```python
from build123d import *

# Parameters (mm, degrees)
SKETCH_1_R      = 2.5
EXTRUDE_1_DEPTH = 90


with BuildPart() as part:
    # 草图1 → 凸台-拉伸1 (new body)
    with BuildSketch(Plane(origin=(0, 0, 0), x_dir=(0, 0, -1), z_dir=(1, 0, 0))):
        with BuildLine():
            Line((10, 8.5), (10, 4))
            ThreePointArc((10, 4), (9.912132034, 3.787867966), (9.7, 3.7))
            ThreePointArc((9.7, 3.7), (9.487867966, 3.612132034), (9.4, 3.4))
            ThreePointArc((9.4, 3.4), (9.312132034, 3.187867966), (9.1, 3.1))
            Line((9.1, 3.1), (8.5, 3.1))
            ThreePointArc((8.5, 3.1), (8.287867966, 3.187867966), (8.2, 3.4))
            Line((8.2, 3.4), (8.2, 5.2))
            ThreePointArc((8.2, 5.2), (8.112132034, 5.412132034), (7.9, 5.5))
            Line((7.9, 5.5), (6.68492424, 5.5))
            ThreePointArc((6.68492424, 5.5), (6.570119211, 5.47716386), (6.472792206, 5.412132034))
            Line((6.472792206, 5.412132034), (4.485786438, 3.425126266))
            ThreePointArc((4.485786438, 3.425126266), (4.052240935, 2.776279568), (3.9, 2.010912703))
            Line((3.9, 2.010912703), (3.9, -2.010912703))
            ThreePointArc((3.9, -2.010912703), (4.052240935, -2.776279568), (4.485786438, -3.425126266))
            Line((4.485786438, -3.425126266), (6.472792206, -5.412132034))
            ThreePointArc((6.472792206, -5.412132034), (6.570119211, -5.47716386), (6.68492424, -5.5))
            Line((6.68492424, -5.5), (7.9, -5.5))
            ThreePointArc((7.9, -5.5), (8.112132034, -5.412132034), (8.2, -5.2))
            Line((8.2, -5.2), (8.2, -3.4))
            ThreePointArc((8.2, -3.4), (8.287867966, -3.187867966), (8.5, -3.1))
            Line((8.5, -3.1), (9.1, -3.1))
            ThreePointArc((9.1, -3.1), (9.312132034, -3.187867966), (9.4, -3.4))
            ThreePointArc((9.4, -3.4), (9.487867966, -3.612132034), (9.7, -3.7))
            ThreePointArc((9.7, -3.7), (9.912132034, -3.787867966), (10, -4))
            Line((10, -4), (10, -8.5))
            ThreePointArc((10, -8.5), (9.560660172, -9.560660172), (8.5, -10))
            Line((8.5, -10), (4, -10))
            ThreePointArc((4, -10), (3.787867966, -9.912132034), (3.7, -9.7))
            ThreePointArc((3.7, -9.7), (3.612132034, -9.487867966), (3.4, -9.4))
            ThreePointArc((3.4, -9.4), (3.187867966, -9.312132034), (3.1, -9.1))
            Line((3.1, -9.1), (3.1, -8.5))
            ThreePointArc((3.1, -8.5), (3.187867966, -8.287867966), (3.4, -8.2))
            Line((3.4, -8.2), (5.2, -8.2))
            ThreePointArc((5.2, -8.2), (5.412132034, -8.112132034), (5.5, -7.9))
            Line((5.5, -7.9), (5.5, -6.68492424))
            ThreePointArc((5.5, -6.68492424), (5.47716386, -6.570119211), (5.412132034, -6.472792206))
            Line((5.412132034, -6.472792206), (3.425126266, -4.485786438))
            ThreePointArc((3.425126266, -4.485786438), (2.776279568, -4.052240935), (2.010912703, -3.9))
            Line((2.010912703, -3.9), (-2.010912703, -3.9))
            ThreePointArc((-2.010912703, -3.9), (-2.776279568, -4.052240935), (-3.425126266, -4.485786438))
            Line((-3.425126266, -4.485786438), (-5.412132034, -6.472792206))
            ThreePointArc((-5.412132034, -6.472792206), (-5.47716386, -6.570119211), (-5.5, -6.68492424))
            Line((-5.5, -6.68492424), (-5.5, -7.9))
            ThreePointArc((-5.5, -7.9), (-5.412132034, -8.112132034), (-5.2, -8.2))
            Line((-5.2, -8.2), (-3.4, -8.2))
            ThreePointArc((-3.4, -8.2), (-3.187867966, -8.287867966), (-3.1, -8.5))
            Line((-3.1, -8.5), (-3.1, -9.1))
            ThreePointArc((-3.1, -9.1), (-3.187867966, -9.312132034), (-3.4, -9.4))
            ThreePointArc((-3.4, -9.4), (-3.612132034, -9.487867966), (-3.7, -9.7))
            ThreePointArc((-3.7, -9.7), (-3.787867966, -9.912132034), (-4, -10))
            Line((-4, -10), (-8.5, -10))
            ThreePointArc((-8.5, -10), (-9.560660172, -9.560660172), (-10, -8.5))
            Line((-10, -8.5), (-10, -4))
            ThreePointArc((-10, -4), (-9.912132034, -3.787867966), (-9.7, -3.7))
            ThreePointArc((-9.7, -3.7), (-9.487867966, -3.612132034), (-9.4, -3.4))
            ThreePointArc((-9.4, -3.4), (-9.312132034, -3.187867966), (-9.1, -3.1))
            Line((-9.1, -3.1), (-8.5, -3.1))
            ThreePointArc((-8.5, -3.1), (-8.287867966, -3.187867966), (-8.2, -3.4))
            Line((-8.2, -3.4), (-8.2, -5.2))
            ThreePointArc((-8.2, -5.2), (-8.112132034, -5.412132034), (-7.9, -5.5))
            Line((-7.9, -5.5), (-6.68492424, -5.5))
            ThreePointArc((-6.68492424, -5.5), (-6.570119211, -5.47716386), (-6.472792206, -5.412132034))
            Line((-6.472792206, -5.412132034), (-4.485786438, -3.425126266))
            ThreePointArc((-4.485786438, -3.425126266), (-4.052240935, -2.776279568), (-3.9, -2.010912703))
            Line((-3.9, -2.010912703), (-3.9, 2.010912703))
            ThreePointArc((-3.9, 2.010912703), (-4.052240935, 2.776279568), (-4.485786438, 3.425126266))
            Line((-4.485786438, 3.425126266), (-6.472792206, 5.412132034))
            ThreePointArc((-6.472792206, 5.412132034), (-6.570119211, 5.47716386), (-6.68492424, 5.5))
            Line((-6.68492424, 5.5), (-7.9, 5.5))
            ThreePointArc((-7.9, 5.5), (-8.112132034, 5.412132034), (-8.2, 5.2))
            Line((-8.2, 5.2), (-8.2, 3.4))
            ThreePointArc((-8.2, 3.4), (-8.287867966, 3.187867966), (-8.5, 3.1))
            Line((-8.5, 3.1), (-9.1, 3.1))
            ThreePointArc((-9.1, 3.1), (-9.312132034, 3.187867966), (-9.4, 3.4))
            ThreePointArc((-9.4, 3.4), (-9.487867966, 3.612132034), (-9.7, 3.7))
            ThreePointArc((-9.7, 3.7), (-9.912132034, 3.787867966), (-10, 4))
            Line((-10, 4), (-10, 8.5))
            ThreePointArc((-10, 8.5), (-9.560660172, 9.560660172), (-8.5, 10))
            Line((-8.5, 10), (-4, 10))
            ThreePointArc((-4, 10), (-3.787867966, 9.912132034), (-3.7, 9.7))
            ThreePointArc((-3.7, 9.7), (-3.612132034, 9.487867966), (-3.4, 9.4))
            ThreePointArc((-3.4, 9.4), (-3.187867966, 9.312132034), (-3.1, 9.1))
            Line((-3.1, 9.1), (-3.1, 8.5))
            ThreePointArc((-3.1, 8.5), (-3.187867966, 8.287867966), (-3.4, 8.2))
            Line((-3.4, 8.2), (-5.2, 8.2))
            ThreePointArc((-5.2, 8.2), (-5.412132034, 8.112132034), (-5.5, 7.9))
            Line((-5.5, 7.9), (-5.5, 6.68492424))
            ThreePointArc((-5.5, 6.68492424), (-5.47716386, 6.570119211), (-5.412132034, 6.472792206))
            Line((-5.412132034, 6.472792206), (-3.425126266, 4.485786438))
            ThreePointArc((-3.425126266, 4.485786438), (-2.776279568, 4.052240935), (-2.010912703, 3.9))
            Line((-2.010912703, 3.9), (2.010912703, 3.9))
            ThreePointArc((2.010912703, 3.9), (2.776279568, 4.052240935), (3.425126266, 4.485786438))
            Line((3.425126266, 4.485786438), (5.412132034, 6.472792206))
            ThreePointArc((5.412132034, 6.472792206), (5.47716386, 6.570119211), (5.5, 6.68492424))
            Line((5.5, 6.68492424), (5.5, 7.9))
            ThreePointArc((5.5, 7.9), (5.412132034, 8.112132034), (5.2, 8.2))
            Line((5.2, 8.2), (3.4, 8.2))
            ThreePointArc((3.4, 8.2), (3.187867966, 8.287867966), (3.1, 8.5))
            Line((3.1, 8.5), (3.1, 9.1))
            ThreePointArc((3.1, 9.1), (3.187867966, 9.312132034), (3.4, 9.4))
            ThreePointArc((3.4, 9.4), (3.612132034, 9.487867966), (3.7, 9.7))
            ThreePointArc((3.7, 9.7), (3.787867966, 9.912132034), (4, 10))
            Line((4, 10), (8.5, 10))
            ThreePointArc((8.5, 10), (9.560660172, 9.560660172), (10, 8.5))
        make_face()
        with Locations(Location((0, 0, 0), (0, 0, 180))):
            Circle(SKETCH_1_R, mode=Mode.SUBTRACT)
    extrude(amount=EXTRUDE_1_DEPTH)


solid = part.part
```
Check sheet for the modelled part. Datum: model origin and axes. Units: mm. A direction names the side the tool comes from. Coordinates: 2 decimals unless noted, no trailing zeros. Write each loop counter-clockwise with the first axis right and the second up, starting at its lowest first coordinate (ties: lowest second). Pieces come first, ordered by that corner, then holes. Notation, with made-up numbers: (21.25, 89) -> (30.25, 89) arc R35 cw to (30.25, 122) -> close; hole circle Ø10 at (48.25, -0.75). An arc over 180 degrees is marked (long way). Use a Markdown table: item, result.
1. Tool access check on faces 4 (the flat face through (44, 0, -3.9)), 5 (the flat face through (44, 8.2, 4)), 6 (the flat face through (44, -3.9, 0)), 7 (the flat face through (44, 3.9, 0)). Record the directions out of +Z, -Z, +X, -X, +Y, -Y that give a thin tool (end or side, any length) a straight path to the whole face; none if there is none.
Reported:
| item | result |
|---|---|
| face 4 | -Z, +X, -X |
| face 5 | +X, -X |
| face 6 | +X, -X, -Y |
| face 7 | +X, -X, +Y |
2. Sectioned sample at A-A (y = 0). Enter the section's corners in (x, z).
Reported:
| item | result |
|---|---|
| outline | (0, -3.9) -> (90, -3.9) -> (90, -2.5) -> (0, -2.5) -> close; (0, 2.5) -> (90, 2.5) -> (90, 3.9) -> (0, 3.9) -> close |
3. Scan lines: line 1 along Y through (x, z) = (26.5, 0); line 2 along Y through (x, z) = (45.5, 8.5); line 3 along Z through (x, y) = (12, 3.5). Record each from-to range of solid material in increasing order.
Reported:
| item | result |
|---|---|
| line 1 | y = -3.9 to -2.5, 2.5 to 3.9 |
| line 2 | y = -10 to -3.1, 3.1 to 10 |
| line 3 | z = -9.42 to -8.2, -4.56 to 4.56, 8.2 to 9.42 |
4. Go/stop test with flat-tipped pins: pin 1 Ø1.2 at (x, z) = (62, 0) entering from +Y; pin 2 Ø3 at (x, z) = (44, 1) entering from -Y; pin 3 Ø0.5 at (x, z) = (55, 9) entering from +Y; pin 4 Ø8 at (y, z) = (0, 0) entering from -X. Record where each tip stops, or that it passes through.
Reported:
| item | result |
|---|---|
| pin 1 | stops at y = 3.9 |
| pin 2 | stops at y = -3.96 |
| pin 3 | stops at y = 9.98 |
| pin 4 | stops at x = 0 |
5. Release check for a two-part mould opening along Y. For faces 1 (the cylindrical face through (44.37, 9.57, -9.55)), 2 (the flat face through (44, -6, 10)), 3 (the cylindrical face through (44.4, -0.1, -2.5)) record: pulls with the +Y half, pulls with the -Y half, needs draft (parallel to the pull), parting line crosses it, or undercut.
Reported:
| item | result |
|---|---|
| face 1 | pulls with the +Y half |
| face 2 | needs draft |
| face 3 | undercut |
